Geometry check sheet. Reference: the model listing, model coordinates, mm. Face numbers are marked on the shaded views. A direction names the side the tool comes from. Coordinates: 2 decimals unless noted, no trailing zeros. Order: outer loops, then holes, each group sorted by start corner. A loop starts at its lowest first (then second) coordinate and runs counter-clockwise, first axis right, second up. Notation, with made-up numbers: (58.25, -14) - (104.25, -14) arc R30 ccw to (104.25, 13) - close; hole circle Ø1 at (38.5, 18). An arc over 180 degrees is marked (long way). Use CSV: the item, a comma, the result in double quotes. Start each with the question number.
1) Sectioned sample at B-B, the plane y = -50.5. Record the cut outline in (x, z), and give its area (3 significant figures).
2) Tool access check on the marked faces 4 and 5. Record the directions out of +Z, -Z, +X, -X, +Y, -Y that give a thin tool (end or side, any length) a straight path to the whole face; none if there is none.
3) Thickness scan on probe 1 along X at (y, z) = (-25.5, 36); probe 2 along Y at (x, z) = (-58, 41.5); probe 3 along Y at (x, z) = (30, 33). Record the ranges inside material, lowest first. Write a range as [from, to].
4) Sectioned sample at A-A, the plane z = 42. Record the cut outline in (x, y).
5) Depth check by flat-ended pin: P1, Ø1, axis at x = -13, y = -43, coming from the +Z side. Enter the tip coordinate at first touch or a pass-through.
6) Draft check along X on the marked faces 1, 2 and 3. Enter one of: released by +X, released by -X, zero draft, split by the parting line, or undercut.
7) Sectioned sample at C-C, the plane z = 25. Record the cut outline in (x, y), and give its area (3 significant figures).
8) Sectioned sample at D-D, the plane x = 4.5. Record the cut outline in (y, z).
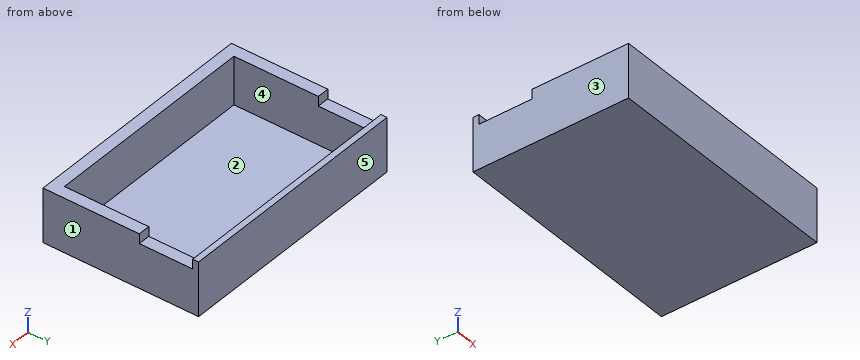
from build123d import *

# Parameters (mm, degrees)
F0_W      = 200
F0_H      = 130
F1_DEPTH  = 5
F2_W      = 200
F2_H      = 10
F3_DEPTH  = 32
F4_W      = 200
F4_H      = 5
F5_DEPTH  = 8
F6_W      = 10
F6_H      = 120
F7_DEPTH  = 32
F8_W      = 10
F8_H      = 120
F9_DEPTH  = 32
F10_W     = 180
F10_H     = 10
F11_DEPTH = 40
F12_W     = 10
F12_H     = 80.5
F13_DEPTH = 8
F14_W     = 10
F14_H     = 80.5
F15_DEPTH = 8


with BuildPart() as f1:
    # F0 (on Top) → F1 (new body)
    with BuildSketch(Plane.XY):
        Rectangle(F0_W, F0_H)
    extrude(amount=F1_DEPTH)

    # F2 (on face) → F3 (join)
    with BuildSketch(Plane.XY.offset(5)):
        with Locations((0, 60)):
            Rectangle(F2_W, F2_H)
    extrude(amount=F3_DEPTH)

    # F4 (on face) → F5 (join)
    with BuildSketch(Plane.XY.offset(37)):
        with Locations((0, 62.5)):
            Rectangle(F4_W, F4_H)
    extrude(amount=F5_DEPTH)

    # F6 (on face) → F7 (join)
    with BuildSketch(Plane.XY.offset(5)):
        with Locations((-95, -5)):
            Rectangle(F6_W, F6_H)
    extrude(amount=F7_DEPTH)

    # F8 (on face) → F9 (join)
    with BuildSketch(Plane.XY.offset(5)):
        with Locations((95, -5)):
            Rectangle(F8_W, F8_H)
    extrude(amount=F9_DEPTH)

    # F10 (on face) → F11 (join)
    with BuildSketch(Plane.XY.offset(5)):
        with Locations((0, -60)):
            Rectangle(F10_W, F10_H)
    extrude(amount=F11_DEPTH)

    # F12 (on face) → F13 (join)
    with BuildSketch(Plane.XY.offset(37)):
        with Locations((95, -24.75)):
            Rectangle(F12_W, F12_H)
    extrude(amount=F13_DEPTH)

    # F14 (on face) → F15 (join)
    with BuildSketch(Plane.XY.offset(37)):
        with Locations((-95, -24.75)):
            Rectangle(F14_W, F14_H)
    extrude(amount=F15_DEPTH)


solid = f1.part
Evaluation:
1,outline,"(-100, 0) - (100, 0) - (100, 45) - (90, 45) - (90, 5) - (-90, 5) - (-90, 45) - (-100, 45) - close"
1,area,"1,800 mm²"
2,face 4,"+Z"
2,face 5,"+Z, -Z, +X, -X, +Y"
3,probe 1,"[-100, -90], [90, 100]"
3,probe 2,"[-65, -55], [60, 65]"
3,probe 3,"[-65, -55], [55, 65]"
4,outline,"(-100, -65) - (100, -65) - (100, 15.5) - (90, 15.5) - (90, -55) - (-90, -55) - (-90, 15.5) - (-100, 15.5) - close; (-100, 60) - (100, 60) - (100, 65) - (-100, 65) - close"
5,P1,"z = 5"
6,face 1,"released by +X"
6,face 2,"undercut"
6,face 3,"released by -X"
7,outline,"(-100, -65) - (100, -65) - (100, 65) - (-100, 65) - close; hole (-90, -55) - (90, -55) - (90, 55) - (-90, 55) - close"
7,area,"6,200 mm²"
8,outline,"(-65, 0) - (65, 0) - (65, 45) - (60, 45) - (60, 37) - (55, 37) - (55, 5) - (-55, 5) - (-55, 45) - (-65, 45) - close"
